The model under review builds one solid part; all positions refer to its coordinate system, in mm. A direction names the side the tool comes from. Give positions to 0.01 mm unless a question says otherwise; leave off trailing zeros. Loops run counter-clockwise (first coordinate to the right, second up) from the corner with the lowest first, then second, coordinate; pieces in that order, holes last. Notation, with made-up numbers: (17, -23.5) - (75, -23.5) arc R24 ccw to (75, 14.5) - close; hole circle Ø4 at (31, 38.25). An arc over 180 degrees is marked (long way). Return JSON: item names as keys, results as strings. Group by question number.
Autodesk Inventor part; units mm, degrees
ref_plane "YZ Plane" through (0, 0, 0) normal (1, 0, 0) x (0, 1, 0)
ref_plane "XZ Plane" through (0, 0, 0) normal (0, 1, 0) x (-1, 0, 0)
ref_plane "XY Plane" through (0, 0, 0) normal (0, 0, 1) x (1, 0, 0)
sketch "Sketch1" plane through (0, 0, 0) normal (0, 0, 1) x (1, 0, 0)
  circle A0 centre (0, 0) radius 1.5
  line L0 (-3, 2) -> (3, 2)
  line L1 (3, 2) -> (3, -2)
  line L2 (3, -2) -> (-3, -2)
  line L3 (-3, -2) -> (-3, 2)
  point P0 (-3, 0)
  point P1 (0, 2)
  dimension "d0" = 3
  dimension "d1" = 6
  dimension "d2" = 4
extrude "Extrusion1" add sketch "Sketch1" along normal blind 2
sketch "Sketch2" plane through (-3, 2, 0) normal (0, 1, 0) x (1, 0, 0)
  line L0 (6, -2) -> (0, -2)
  line L1 (1.75, -2) -> (4.25, -2)
  line L2 (4.25, -2) -> (4.25, -5)
  line L3 (4.25, -5) -> (1.75, -5)
  line L4 (1.75, -5) -> (1.75, -2)
  line L5 (-0.0919, -3.875) -> (-1.0919, -3.875)
  line L6 (-1.0919, -3.875) -> (-1.0919, -8.875)
  line L7 (-1.0919, -8.875) -> (-0.0919, -8.875)
  line L8 (-0.0919, -8.875) -> (-0.0919, -3.875)
  line L9 (-0.5919, -3.875) -> (1.75, -2) construction
  line L10 (1.75, -2) -> (2.25, -2.6245) construction
  line L11 (2.25, -2.6245) -> (-0.0919, -4.4995) construction
  line L12 (-0.0919, -4.4995) -> (-0.5919, -3.875) construction
  line L13 (-0.0919, -6.375) -> (2.3038, -4.0774) construction
  line L14 (2.3038, -4.0774) -> (1.75, -3.5) construction
  line L15 (1.75, -3.5) -> (-0.6456, -5.7976) construction
  line L16 (-0.6456, -5.7976) -> (-0.0919, -6.375) construction
  line L17 (6.0919, -8.875) -> (7.0919, -8.875)
  line L18 (7.0919, -8.875) -> (7.0919, -3.875)
  line L19 (7.0919, -3.875) -> (6.0919, -3.875)
  line L20 (6.0919, -3.875) -> (6.0919, -8.875)
  line L21 (4.25, -2) -> (6.5919, -3.875) construction
  line L22 (6.5919, -3.875) -> (6.0919, -4.4995) construction
  line L23 (6.0919, -4.4995) -> (3.75, -2.6245) construction
  line L24 (3.75, -2.6245) -> (4.25, -2) construction
  line L25 (6.0919, -6.375) -> (3.6962, -4.0774) construction
  line L26 (3.6962, -4.0774) -> (4.25, -3.5) construction
  line L27 (4.25, -3.5) -> (6.6456, -5.7976) construction
  line L28 (6.6456, -5.7976) -> (6.0919, -6.375) construction
  line L29 (-0.0919, -6.375) -> (1.75, -4.6085)
  line L30 (-0.0919, -6.375) -> (-0.0919, -5.2665)
  line L31 (-0.0919, -5.2665) -> (1.75, -3.5)
  line L32 (1.75, -3.5) -> (1.75, -4.6085)
  line L33 (-0.0919, -4.4995) -> (-0.0919, -3.875)
  line L34 (-0.0919, -3.875) -> (-0.5919, -3.875)
  line L35 (-0.5919, -3.875) -> (1.75, -2)
  line L36 (1.75, -2) -> (1.75, -3.0248)
  line L37 (1.75, -3.0248) -> (-0.0919, -4.4995)
  line L38 (6.0919, -6.375) -> (6.0919, -5.2665)
  line L39 (6.0919, -5.2665) -> (4.25, -3.5)
  line L40 (4.25, -3.5) -> (4.25, -4.6085)
  line L41 (4.25, -4.6085) -> (6.0919, -6.375)
  line L42 (4.25, -3.0248) -> (6.0919, -4.4995)
  line L43 (6.0919, -4.4995) -> (6.0919, -3.875)
  line L44 (6.0919, -3.875) -> (6.5919, -3.875)
  line L45 (6.5919, -3.875) -> (4.25, -2)
  line L46 (4.25, -2) -> (4.25, -3.0248)
  point P0 (3, 0)
  point P1 (3, -2)
  dimension "d5" = 2.5
  dimension "d6" = 3
  dimension "d7" = 1
  dimension "d8" = 5
  dimension "d11" = 0.8
  dimension "d13" = 3
  dimension "d15" = 0.8
  dimension "d18" = 1
  dimension "d19" = 5
  dimension "d20" = 0.8
  dimension "d21" = 3
  dimension "d22" = 0.8
extrude "Extrusion3" add sketch "Sketch2" against normal blind 4 contours L2 L3 L4 L0 | L45 L19 L20 L42 L2 | L4 L37 L8 L5 L35 | L19 L18 L17 L20 | L5 L8 L7 L6 | L39 L20 L41 L2 | L4 L29 L8 L31
fillet "Fillet1" radius 1 6 edges at (-4.0919, 0, 8.875) (4.0919, 0, 8.875) (4.0919, 0, 3.875) (-4.0919, 0, 3.875) (-1.25, 0, 5) (1.25, 0, 5)
sketch "Sketch5" plane through (-3, 2, 0) normal (0, 1, 0) x (1, 0, 0)
  line L0 (1.75, -2) -> (0, -2)
  line L1 (0, -2) -> (0, -3.4011)
  line L2 (1.75, -2) -> (-0.5919, -3.875)
  line L3 (1.75, -2) -> (0, -3.4011)
  line L4 (6, -2) -> (6, -3.4011)
  line L5 (4.25, -2) -> (1.75, -2)
  line L6 (6, -3.4011) -> (4.25, -2)
  line L7 (4.25, -2) -> (6, -2)
  line L8 (6.5919, -3.875) -> (4.25, -2)
  point P0 (3, 0)
extrude "Extrusion4" add sketch "Sketch5" against normal blind 4
sketch "Sketch6" plane through (0, 0, 0) normal (0, 0, -1) x (-1, 0, 0)
  circle A0 centre (0, 0) radius 1.5
extrude "Extrusion5" cut sketch "Sketch6" against normal through all
sketch "Sketch7" plane through (-0.4564, 2, 5) normal (0, 0, 1) x (1, 0, 0)
  circle A0 centre (0.4564, -2) radius 3
  dimension "d31" = 6
extrude "Extrusion6" cut sketch "Sketch7" along normal mid plane 4
properties part number "Arm8" material "ABS Plastic"
Item 1: Mouldability with a two-part tool opening along X and no side actions: class faces 4 (the face through (3.79, 0.03, 8.59)), 5 (the face through (3, 0, 4)), 6 (the face through (0, -2, 2)), 7 (the face through (-3, 0, 2)) as +X half, -X half, draft (parallel to the pull), parting line (faces both ways), or undercut.
Item 2: For L1, parallel to X at y = 0, z = 2.5; L2, parallel to Y at x = 0, z = 2.2; L3, parallel to X at y = 1.3, z = 7.5, list the stretches that pass through material, from the lowest coordinate up. Write a range as from..to.
Item 3: Take a section at B-B (x = 0). State the section outline as (y, z) points, then the cut area to 3 significant figures.
Item 4: Take a section at A-A (z = 8). State the section outline as (x, y) points.
Item 5: Tool access review of faces 1 (the face through (-3, 0, 6)), 2 (the face through (-3.81, 0.03, 8.57)), 3 (the face through (3, 0, 2)): name each direction out of +Z, -Z, +X, -X, +Y, -Y from which nothing blocks a thin tool from reaching the whole face with its end or side.
Item 6: For P1, Ø1.5, axis at x = 1.5, y = 1, coming from the +Z side; P2, Ø1, axis at x = 1.5, y = 1, coming from the -Z side; P3, Ø1, axis at y = -0.5, z = 1.5, coming from the -X side, all flat-tipped, find the tip position at first contact; note any pin that passes through.
Item 7: Take a section at D-D (z = 1). State the section outline as (x, y) points.
Check sheet entries:
{
 "1": {"face 4": "+X half", "face 5": "undercut", "face 6": "draft", "face 7": "-X half"},
 "2": {"L1": "x = -3..-1.5, 1.5..3", "L2": "y = -2..-1.5, 1.5..2", "L3": "x = -4.09..-3.09, 3.09..4.09"},
 "3": {"outline": "(-2, 0) - (-1.5, 0) - (-1.5, 3) - (-2, 3) - close; (1.5, 0) - (2, 0) - (2, 3) - (1.5, 3) - close", "area": "3.00 mm^2"},
 "4": {"outline": "(-4.08, -2) - (-3.09, -2) - (-3.09, 2) - (-4.08, 2) - close; (3.09, -2) - (4.08, -2) - (4.08, 2) - (3.09, 2) - close"},
 "5": {"face 1": "+Z", "face 2": "+Z, -X, +Y, -Y", "face 3": "-Z, +X, +Y, -Y"},
 "6": {"P1": "stops at z = 3", "P2": "stops at z = 0", "P3": "stops at x = -3"},
 "7": {"outline": "(-3, -2) - (3, -2) - (3, 2) - (-3, 2) - close; hole circle Ø3 at (0, 0)"}
}
